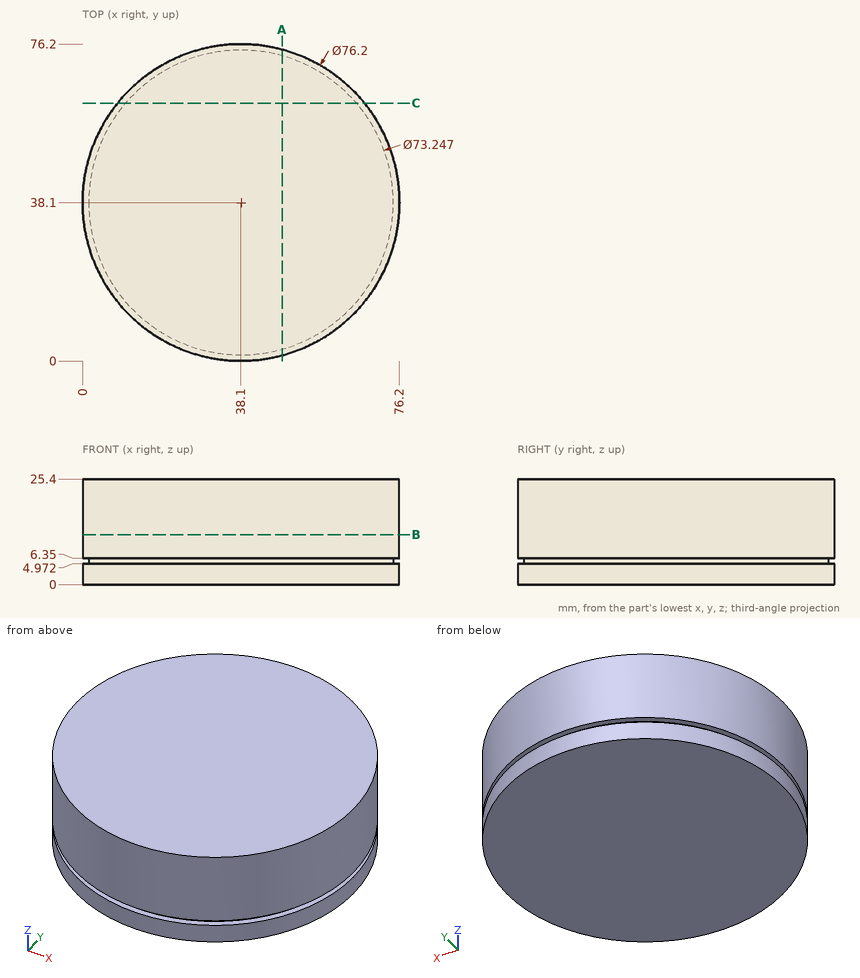
Geometry check sheet. Reference: drawing and pictorial views, mm from the part's lowest x, y, z. Round coordinates to 2 decimals unless told otherwise and drop trailing zeros. Order: outer loops, then holes, each group sorted by start corner. A loop starts at its lowest first (then second) coordinate and runs counter-clockwise, first axis right, second up. Notation, with made-up numbers: M 36.25,61.25 L 92.25,61.25 A22 ccw 92.25,89.25 Z; hole C 71.25,34.25 d9. An arc over 180 degrees is marked long. Answer as CSV lines item,"result".
1) Gauge pin test, flat ends, axial feed: pin 1 Ø6 at (x, z) = (45.5, 17.5) entering from -Y (3 decimals); pin 2 Ø5 at (x, z) = (62.5, 22) entering from +Y; pin 3 Ø4 at (y, z) = (49.5, 18.5) entering from -X. Record the tip position at first contact, or that the pin passes through.
Entries:
pin 1,"y = 0.255"
pin 2,"y = 69.28"
pin 3,"x = 1.18"
2) Sectioned sample at B-B on z = 12. Record the cut outline in (x, y), and give its area (3 significant figures).
Entries:
outline,"C 38.1,38.1 d76.2"
area,"4,560 mm2"
3) Thickness scan on probe 1 along X at (y, z) = (53, 14.25) (1 decimal); probe 2 along X at (y, z) = (27, 15); probe 3 along Y at (x, z) = (5, 16.5). Record the ranges inside material, lowest first. Write a range as [from, to].
Entries:
probe 1,"[3, 73.2]"
probe 2,"[1.65, 74.55]"
probe 3,"[19.23, 56.97]"
4) Sectioned sample at C-C on y = 62. Record the cut outline in (x, z), and give its area (3 significant figures).
Entries:
outline,"M 8.43,0 L 67.77,0 L 67.77,4.97 L 65.85,4.97 L 65.85,6.35 L 67.77,6.35 L 67.77,25.4 L 8.43,25.4 L 8.43,6.35 L 10.35,6.35 L 10.35,4.97 L 8.43,4.97 Z"
area,"1,500 mm2"
5) Sectioned sample at A-A on x = 48. Record the cut outline in (y, z), and give its area (3 significant figures).
Entries:
outline,"M 1.31,0 L 74.89,0 L 74.89,4.97 L 73.36,4.97 L 73.36,6.35 L 74.89,6.35 L 74.89,25.4 L 1.31,25.4 L 1.31,6.35 L 2.84,6.35 L 2.84,4.97 L 1.31,4.97 Z"
area,"1,860 mm2"
